The model under review builds one solid part; all positions refer to its coordinate system, in mm. A direction names the side the tool comes from. Give positions to 0.01 mm unless a question says otherwise; leave off trailing zeros. Loops run counter-clockwise (first coordinate to the right, second up) from the corner with the lowest first, then second, coordinate; pieces in that order, holes last. Notation, with made-up numbers: M 12,42.25 L 23,42.25 A31 ccw 23,78.25 Z; hole C -3.75,-22 d1. An arc over 180 degrees is marked long. One line per item, written item: value. Start each with the question number.
Q1. We need section C-C on y = 40. Write out the cut boundary in (x, z), plus the area to 3 significant figures.
Q2. We need section A-A on x = 0. Write out the cut boundary in (y, z), plus the area to 3 significant figures.
Q3. We need section B-B on z = 0. Write out the cut boundary in (x, y).
Q4. We need section D-D on z = -36. Write out the cut boundary in (x, y), plus the area to 3 significant figures.
Q5. To check wall thickness, follow line 1 along X through (y, z) = (70, -53); line 2 along Y through (x, z) = (116, 23); line 3 along Z through (x, y) = (-38.5, 73.5). State the ranges of each line that lie inside material, in increasing order. Write a range as from..to.
Q6. Mouldability with a two-part tool opening along Z and no side actions: class faces 1 (the face through (46, 20, 105)), 2 (the face through (46.08, 80.25, -11.49)), 3 (the face through (-47.75, 80.25, -11.49)), 4 (the face through (46, 55, -90.04)) as released by +Z, released by -Z, zero draft, split by the parting line, or undercut.
Q7. For pin 1 (2 mm diameter, centred on y = 12, z = -75, fed in from -X); pin 2 (1 mm diameter, centred on y = 43, z = -70.5, fed in from -X); pin 3 (8 mm diameter, centred on y = 12.5, z = -21, fed in from -X), all flat-tipped, find the tip position at first contact; note any pin that passes through.
Q8. For faces 5 (the face through (63.982, 35, 27)), 6 (the face through (46, 20, -105)), 7 (the face through (-92, 15, -2)), 8 (the face through (-2, 5, 95)), list the 3-axis set-ups (+Z, -Z, +X, -X, +Y, -Y) from which the entire face can be reached by the end or side of a thin tool; tool diameter is ignored.
```python
from build123d import *

# Parameters (mm, degrees)
SKETCH2_R           = 132
BOSS_EXTRUDE1_DEPTH = 90
SKETCH3_W           = 57.679416137
SKETCH3_H           = 85
CUT_EXTRUDE1_DEPTH  = 160
SKETCH4_W           = 66
SKETCH4_H           = 75
SKETCH4_W_2         = 69.873766725
SKETCH4_H_2         = 74.92536342
CUT_EXTRUDE2_DEPTH  = 160
SKETCH5_R           = 30
CUT_EXTRUDE3_DEPTH  = 160
SKETCH6_W           = 57.679416137
SKETCH6_H           = 128.655011674
CUT_EXTRUDE4_DEPTH  = 160
SKETCH7_W           = 202.247474543
SKETCH7_H           = 277.255171559
SKETCH7_W_2         = 143.334546523
SKETCH7_H_2         = 180
CUT_EXTRUDE5_DEPTH  = 70


with BuildPart() as part:
    # Sketch2 → Boss-Extrude1 (new body)
    with BuildSketch(Plane(origin=(0, 0, 0), x_dir=(1, 0, 0), z_dir=(0, 1, 0))):
        with Locations(Location((0, 0, 0), (0, 0, 90))):
            Circle(SKETCH2_R)
    extrude(amount=BOSS_EXTRUDE1_DEPTH)

    # Sketch3 → Cut-Extrude1 (cut, symmetric)
    with BuildSketch(Plane.XY):
        with Locations((-1.160291932, 47.5)):
            Rectangle(SKETCH3_W, SKETCH3_H)
    extrude(amount=CUT_EXTRUDE1_DEPTH, both=True, mode=Mode.SUBTRACT)

    # Sketch4 → Cut-Extrude2 (cut, symmetric)
    with BuildSketch(Plane.XY):
        with Locations((-99, 52.5)):
            Rectangle(SKETCH4_W, SKETCH4_H)
        with Locations((98.918931808, 52.53731829)):
            Rectangle(SKETCH4_W_2, SKETCH4_H_2)
    extrude(amount=CUT_EXTRUDE2_DEPTH, both=True, mode=Mode.SUBTRACT)

    # Sketch5 → Cut-Extrude3 (cut, symmetric)
    with BuildSketch(Plane(origin=(63.982048445, 0, 0), x_dir=(0, 0, -1), z_dir=(1, 0, 0))):
        with Locations(Location((0, 52.53731829, 0), (0, 0, 90))):
            Circle(SKETCH5_R)
    extrude(amount=CUT_EXTRUDE3_DEPTH, both=True, mode=Mode.SUBTRACT)

    # Sketch6 → Cut-Extrude4 (cut, symmetric)
    with BuildSketch(Plane(origin=(0, 5, 0), x_dir=(1, 0, 0), z_dir=(0, 1, 0))):
        with Locations((-1.160291932, 7.462587684)):
            Rectangle(SKETCH6_W, SKETCH6_H)
    extrude(amount=CUT_EXTRUDE4_DEPTH, both=True, mode=Mode.SUBTRACT)

    # Sketch7 → Cut-Extrude5 (cut, symmetric)
    with BuildSketch(Plane(origin=(0, 90, 0), x_dir=(1, 0, 0), z_dir=(0, 1, 0))):
        with Locations((-4.464336864, -2.73307398)):
            Rectangle(SKETCH7_W, SKETCH7_H)
        with Locations((-1.427587997, 0.039603907)):
            Rectangle(SKETCH7_W_2, SKETCH7_H_2, mode=Mode.SUBTRACT)
    extrude(amount=CUT_EXTRUDE5_DEPTH, both=True, mode=Mode.SUBTRACT)


solid = part.part
```
Solved:
1. outline: M -66,-90.04 L -30,-90.04 L -30,-27.25 L -66,-27.25 Z; M -66,27.25 L -30,27.25 L -30,89.96 L -66,89.96 Z; M 27.68,-90.04 L 63.98,-90.04 L 63.98,-27.25 L 27.68,-27.25 Z; M 27.68,27.25 L 63.98,27.25 L 63.98,89.96 L 27.68,89.96 Z
1. area: 9,070 mm2
2. outline: M 0,-132 L 5,-132 L 5,-71.79 L 0,-71.79 Z; M 0,56.86 L 5,56.86 L 5,132 L 0,132 Z
2. area: 677 mm2
3. outline: M -132,0 L -30,0 L -30,22.54 L -66,22.54 L -66,15 L -132,15 Z; M -66,82.54 L -30,82.54 L -30,90 L -66,90 Z; M 27.68,0 L 132,0 L 132,15.07 L 63.98,15.07 L 63.98,22.54 L 27.68,22.54 Z; M 27.68,82.54 L 63.98,82.54 L 63.98,90 L 27.68,90 Z
4. outline: M -127,0 L -30,0 L -30,90 L -66,90 L -66,15 L -127,15 Z; M 27.68,0 L 127,0 L 127,15.07 L 63.98,15.07 L 63.98,90 L 27.68,90 Z
4. area: 8,370 mm2
5. line 1: -66..-30, 27.68..63.98
5. line 2: 0..15.07
5. line 3: -90.04..-21.46, 21.46..89.96
6. face 1: zero draft
6. face 2: undercut
6. face 3: undercut
6. face 4: released by -Z
7. pin 1: x = -109.31
7. pin 2: x = -66
7. pin 3: x = -130.9
8. face 5: +Z, -Z, +X, +Y
8. face 6: -Z, +X, -X, +Y
8. face 7: +Z, -Z, -X, +Y
8. face 8: +Z, -Z, +Y
